Source: three-view drawing plus pictorial views. Frame: mm from the lowest corner of the part. Give positions to 0.01 mm unless a question says otherwise; leave off trailing zeros. Loops run counter-clockwise (first coordinate to the right, second up) from the corner with the lowest first, then second, coordinate; pieces in that order, holes last.
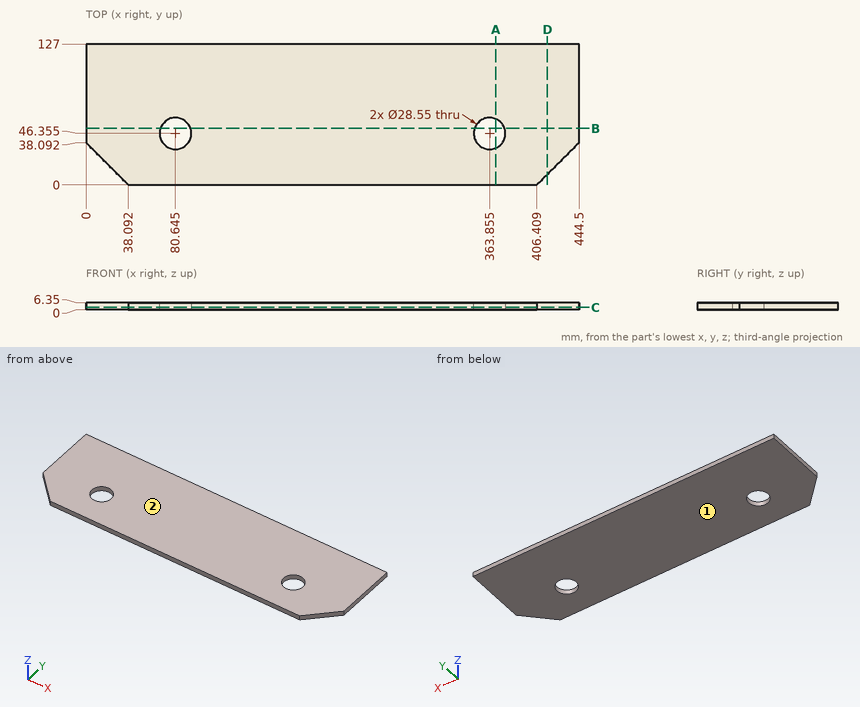
1) Cut plane A-A (x = 369.5). Return loops of the section in (y, z).
Checks:
outline: (0, 0) - (33.24, 0) - (33.24, 6.35) - (0, 6.35) - close; (59.47, 0) - (127, 0) - (127, 6.35) - (59.47, 6.35) - close
2) Cut plane D-D (x = 416). Return loops of the section in (y, z).
Checks:
outline: (9.59, 0) - (127, 0) - (127, 6.35) - (9.59, 6.35) - close
3) Ray query, probe 1 along X at (y, z) = (45, 5.75) (1 decimal); probe 2 along X at (y, z) = (59, 4) (1 decimal); probe 3 along Y at (x, z) = (74, 3). Return the intervals inside material, ascending.
Checks:
probe 1: x = 0 to 66.4, 94.9 to 349.6, 378.1 to 444.5
probe 2: x = 0 to 74, 87.3 to 357.2, 370.5 to 444.5
probe 3: y = 0 to 33.72, 58.99 to 127
4) Pull-direction query (Z, two-part tool) for the marked faces 1 and 2; classes: released by +Z, released by -Z, zero draft, split by the parting line, or undercut.
Checks:
face 1: released by -Z
face 2: released by +Z
5) Cut plane C-C (z = 2.25). State how many separate pieces and enclosed holes the cut face has, and give its area (3 significant figures).
Checks:
separate pieces: 1
enclosed holes: 2
area: 53,700 mm2
6) Cut plane B-B (y = 51). Return loops of the section in (x, z).
Checks:
outline: (0, 0) - (67.15, 0) - (67.15, 6.35) - (0, 6.35) - close; (94.14, 0) - (350.36, 0) - (350.36, 6.35) - (94.14, 6.35) - close; (377.35, 0) - (444.5, 0) - (444.5, 6.35) - (377.35, 6.35) - close
